from build123d import *

# Parameters (mm, degrees)
M12_TAPPED_HOLE1_D           = 10.2
M12_TAPPED_HOLE1_DEPTH       = 16.935610843
M12_TAPPED_HOLE1_CSINK_D     = 12.05
M12_TAPPED_HOLE1_CSINK_ANGLE = 90
M12_TAPPED_HOLE1_TIP         = 3.064389157
FILLET1_R                    = 1
CHAMFER1_SIZE                = 1
SCALE1_SCALE                 = 0.625


with BuildPart() as part:
    # Sketch1 → Revolve1 (revolve)
    with BuildSketch(Plane.XY):
        Polygon((0, 0), (0, 24), (70, 24), (70, 20), (75, 20), (75, 15), (91, 15), (91, 13.95), (92.5, 13.95), (92.5, 15), (100, 15), (100, 0), align=None)
    revolve(axis=Axis((100, 0, 0), (-1, 0, 0)))

    # M12 Tapped Hole1
    with Locations(Plane.ZY):
        with Locations((0, 0)):
            CounterSinkHole(M12_TAPPED_HOLE1_D / 2, M12_TAPPED_HOLE1_CSINK_D / 2, depth=M12_TAPPED_HOLE1_DEPTH, counter_sink_angle=M12_TAPPED_HOLE1_CSINK_ANGLE)
            with Locations((0, 0, -(M12_TAPPED_HOLE1_DEPTH + M12_TAPPED_HOLE1_TIP / 2))):  # 118° drill point
                Cone(0, M12_TAPPED_HOLE1_D / 2, M12_TAPPED_HOLE1_TIP, mode=Mode.SUBTRACT)

    # Fillet1
    fillet1_edges = [part.edges().sort_by_distance(p)[0] for p in [
        (75, -15, 0),
        (70, -20, 0),
    ]]
    fillet(fillet1_edges, radius=FILLET1_R)

    # Chamfer1
    chamfer1_edges = [part.edges().sort_by_distance(p)[0] for p in [
        (75, -20, 0),
        (70, -24, 0),
        (0, -24, 0),
        (100, -15, 0),
    ]]
    chamfer(chamfer1_edges, length=CHAMFER1_SIZE)


with BuildPart() as part_1:
    # Scale1: scaled about (42.999626609, 0, 0)
    add(part.part.scale(SCALE1_SCALE).moved(Location((16.124859978, 0, 0))))

    # Mirror2: part across plane


with BuildPart() as part_2:
    add(part_1.part)
    add(part_1.part.mirror(Plane.ZY.offset(-37.999859978)))


solid = part_2.part
Geometry check sheet. Reference: the model listing, model coordinates, mm. A direction names the side the tool comes from. Coordinates: 2 decimals unless noted, no trailing zeros. Loops run counter-clockwise (first coordinate to the right, second up) from the corner with the lowest first, then second, coordinate; pieces in that order, holes last. Notation, with made-up numbers: (7.5, -7) - (36.5, -7) arc R26 ccw to (36.5, 9) - close; hole circle Ø4 at (-39.75, 54.5). An arc over 180 degrees is marked (long way). Use one line per item in the form item = value. Start each with the question number.
Item 1: Gauge pin test, flat ends, axial feed: pin 1 (2 mm diameter, centred on y = -6, z = 11, fed in from +X); pin 2 (4 mm diameter, centred on y = -9, z = -10, fed in from -X); pin 3 (1.5 mm diameter, centred on x = 20.5, z = 7.5, fed in from +Y). Record the tip position at first contact, or that the pin passes through.
Item 2: Section check B-B, the plane x = 24. Enter the section's corners in (y, z).
Item 3: Section check A-A, the plane x = 7.5. Enter the section's corners in (y, z) (3 decimals).
Item 4: Mould release check, pull along X, two halves, no side actions. Record for faces 4 (the face through (63, -5, 9)), 5 (the face through (16.125, -6, 12)), 6 (the face through (75.997, -1.22, -9.295)), 7 (the face through (2.062, -7, 6)): +X half, -X half, draft (parallel to the pull), parting line (faces both ways), or undercut.
Item 5: Tool access check on faces 1 (the face through (0.003, -1.22, -9.295)), 2 (the face through (2.525, -6.919, 5.305)), 3 (the face through (59.875, 6, 12)). Record the directions out of +Z, -Z, +X, -X, +Y, -Y that give a thin tool (end or side, any length) a straight path to the whole face; none if there is none.
Item 6: Thickness scan on probe 1 along X at (y, z) = (5.25, -12); probe 2 along X at (y, z) = (-9.75, -1.5); probe 3 along X at (y, z) = (-6.5, 6). Record the ranges inside material, lowest first.
Computed:
q1.pin_1 = 63
q1.pin_2 = 13
q1.pin_3 = 13.4
q2.outline = circle Ø30 at (0, 0)
q3.outline = circle Ø18.75 at (0, 0)
q4.face_4 = +X half
q4.face_5 = -X half
q4.face_6 = draft
q4.face_7 = undercut
q5.face_1 = -X
q5.face_2 = none
q5.face_3 = +X
q6.probe_1 = 16.12 to 59.88
q6.probe_2 = 12.99 to 63.01
q6.probe_3 = -2.53 to 2.06, 3 to 73, 73.94 to 78.53
